```python
from build123d import *

# Parameters (mm, degrees)
SKETCH_R           = 50
SKETCH_R_2         = 25
PAD_DEPTH          = 2
SKETCH001_R        = 1
POCKET_DEPTH       = 282.871995
POCKET_DEPTH_BACK  = 284.871995
POLARPATTERN_COUNT = 8


with BuildPart() as part:
    # Sketch → Pad (new body)
    with BuildSketch(Plane.XY):
        Circle(SKETCH_R)
        Circle(SKETCH_R_2, mode=Mode.SUBTRACT)
    extrude(amount=PAD_DEPTH)

    # Sketch001 → Pocket (cut, two sides)
    with BuildSketch(Plane.XY) as pocket_sk:
        with Locations((30, 0)):
            Circle(SKETCH001_R)
        with Locations((45, 0)):
            Circle(SKETCH001_R)
    pocket = extrude(amount=-POCKET_DEPTH, mode=Mode.SUBTRACT) + extrude(pocket_sk.sketch, amount=POCKET_DEPTH_BACK, mode=Mode.SUBTRACT)

    # PolarPattern: Pocket ×8 about axis
    polarpattern_axis = Axis((0, 0, 0), (0, 0, 1))
    for i in range(1, POLARPATTERN_COUNT):
        add(pocket.rotate(polarpattern_axis, i * 360 / POLARPATTERN_COUNT), mode=Mode.SUBTRACT)


solid = part.part
```
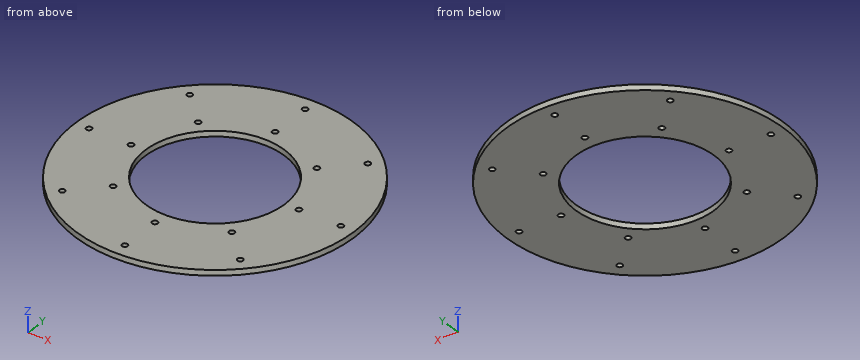
The listing builds one solid part. Answer for the finished solid, in the listing's coordinates (mm). Coordinates: 2 decimals unless noted, no trailing zeros. Loops run counter-clockwise (first coordinate to the right, second up) from the corner with the lowest first, then second, coordinate; pieces in that order, holes last. Notation, with made-up numbers: (26, -35.5) -> (85, -35.5) arc R22 cw to (85, -15.5) -> close; hole circle Ø2 at (78.25, 3). An arc over 180 degrees is marked (long way). Use one line per item in the form item = value. Start each with the question number.
Item 1: The part is cut by section C-C on z = 1.6. Count the separate pieces of the cut face and the enclosed holes in it, then the cut area to 3 significant figures.
Item 2: The part is cut by section B-B on y = -17.5. Determine the outline of the cut face in (x, z), then the cut area to 3 significant figures.
Item 3: The part is cut by section D-D on y = 35.5. Determine the outline of the cut face in (x, z).
Item 4: The part is cut by section A-A on x = -18.5. Determine the outline of the cut face in (y, z), then the cut area to 3 significant figures.
Item 5: Consider L1, parallel to X at y = 20.5, z = 0.55; L2, parallel to Y at x = 2, z = 1.2; L3, parallel to Y at x = -7, z = 0.8. Determine where each line is inside the solid, lowest interval first. Write a range as [from, to].
Answer key:
q1.separate_pieces = 1
q1.enclosed_holes = 17
q1.area = 5,840 mm2
q2.outline = (-46.84, 0) -> (-17.85, 0) -> (-17.85, 2) -> (-46.84, 2) -> close; (17.85, 0) -> (46.84, 0) -> (46.84, 2) -> (17.85, 2) -> close
q2.area = 116 mm2
q3.outline = (-35.21, 0) -> (35.21, 0) -> (35.21, 2) -> (-35.21, 2) -> close
q4.outline = (-46.45, 0) -> (-16.82, 0) -> (-16.82, 2) -> (-46.45, 2) -> close; (16.82, 0) -> (46.45, 0) -> (46.45, 2) -> (16.82, 2) -> close
q4.area = 119 mm2
q5.L1 = [-45.6, -21.91], [-20.51, -14.31], [14.31, 20.51], [21.91, 45.6]
q5.L2 = [-49.96, -24.92], [24.92, 49.96]
q5.L3 = [-49.51, -24], [24, 49.51]
